Verification items for this drawing (mm, ordinates from the low corner). Give positions to 0.01 mm unless a question says otherwise; leave off trailing zeros. Loops run counter-clockwise (first coordinate to the right, second up) from the corner with the lowest first, then second, coordinate; pieces in that order, holes last. Notation, with made-up numbers: (82.25, 86.25) -> (117.25, 86.25) arc R16 ccw to (117.25, 94.25) -> close; hole circle Ø9 at (50.5, 15.5). An arc over 180 degrees is marked (long way). Write each question's results on one line, items separated by ' | '. Start each with the question number.
Item 1: Mould release check, pull along Y, two halves, no side actions. Record for the marked faces 1, 2 and 3: pulls with the +Y half, pulls with the -Y half, needs draft (parallel to the pull), parting line crosses it, or undercut.
Item 2: Cross-section at C-C on z = 20.5. Enter the section's corners in (x, y).
Item 3: Cross-section at A-A on y = 32.5. Enter the section's corners in (x, z).
Item 4: Scan lines: line 1 along Y through (x, z) = (32.5, 22); line 2 along Y through (x, z) = (42, 17.5); line 3 along Z through (x, y) = (37, 44). Record each from-to range of solid material in increasing order.
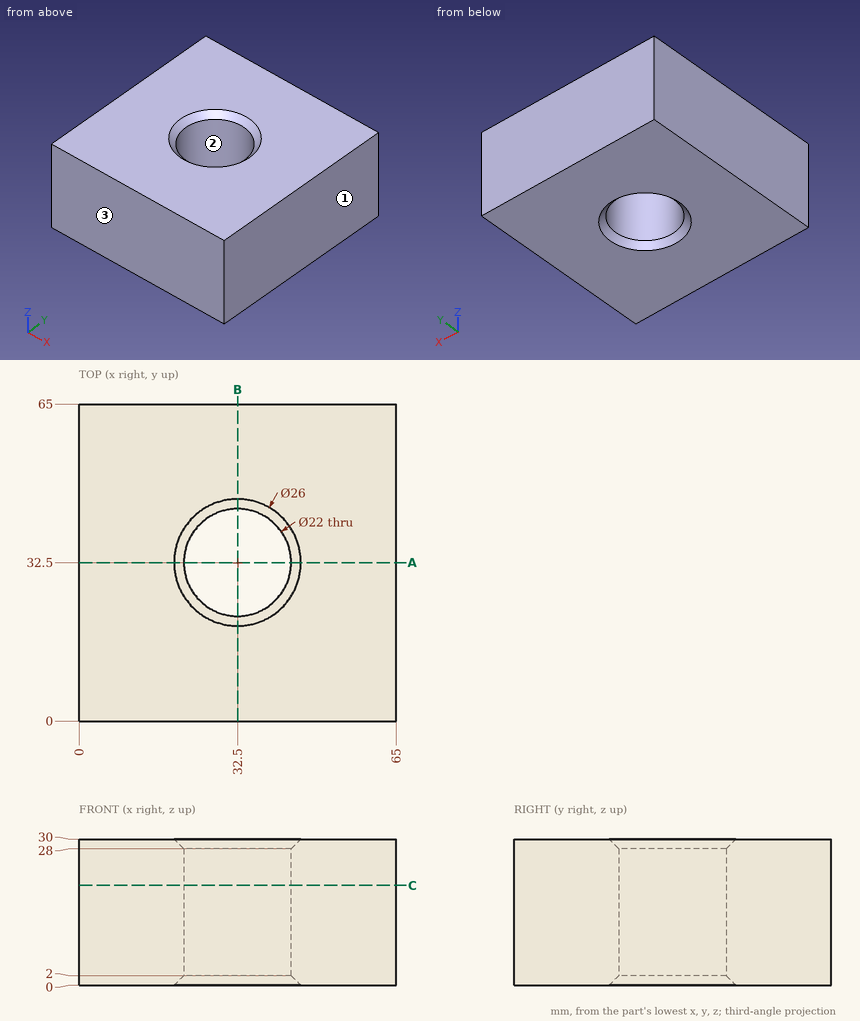
Answer sheet:
1) face 1: needs draft | face 2: undercut | face 3: pulls with the -Y half
2) outline: (0, 0) -> (65, 0) -> (65, 65) -> (0, 65) -> close; hole circle Ø22 at (32.5, 32.5)
3) outline: (0, 0) -> (19.5, 0) -> (21.5, 2) -> (21.5, 28) -> (19.5, 30) -> (0, 30) -> close; (43.5, 2) -> (45.5, 0) -> (65, 0) -> (65, 30) -> (45.5, 30) -> (43.5, 28) -> close
4) line 1: y = 0 to 21.5, 43.5 to 65 | line 2: y = 0 to 26.95, 38.05 to 65 | line 3: z = 0.65 to 29.35
